```python
from build123d import *

# Parameters (mm, degrees)
SKETCH1_W                = 7.9
SKETCH1_H                = 95.7
BOSS_EXTRUDE1_DEPTH      = 9.2
SKETCH1_3_W              = 7.9
SKETCH1_3_H              = 95.7
BOSS_EXTRUDE2_DEPTH      = 9.2
BOSS_EXTRUDE3_DEPTH      = 32
BOSS_EXTRUDE3_DEPTH_BACK = 16
SKETCH2_R                = 3.8
BOSS_EXTRUDE4_DEPTH      = 0.0001
BOSS_EXTRUDE4_DEPTH_BACK = 6
SKETCH4_R                = 0.5


with BuildPart() as part:
    # Sketch1 → Boss-Extrude1 (new body)
    with BuildSketch(Plane(origin=(0, 0, 0), x_dir=(0, 0, -1), z_dir=(1, 0, 0))):
        with Locations((-28.171698113, -0.670754717)):
            Rectangle(SKETCH1_W, SKETCH1_H)
    extrude(amount=BOSS_EXTRUDE1_DEPTH)

    # Sketch1_3 → Boss-Extrude2 (add)
    with BuildSketch(Plane(origin=(0, 0, 0), x_dir=(0, 0, -1), z_dir=(1, 0, 0))):
        with Locations((-28.171698113, -0.670754717)):
            Rectangle(SKETCH1_3_W, SKETCH1_3_H)
        with Locations((-4.071698113, -0.670754717)):
            Rectangle(SKETCH1_3_W, SKETCH1_3_H)
    extrude(amount=BOSS_EXTRUDE2_DEPTH)


with BuildPart() as boss_extrude2_piece_1:
    # of the separate pieces the step leaves, piece 1, a body of its own (boss_extrude2_pieces)
    add(part.part.solids().sort_by_distance((0, 47.179245283, 8.021698113))[0])



with BuildPart() as boss_extrude2_piece_2:
    # of the separate pieces the step leaves, piece 2, a body of its own (boss_extrude2_pieces)
    add(part.part.solids().sort_by_distance((0, 47.179245283, 32.121698113))[0])


with BuildPart() as boss_extrude2_piece_1_1:
    add(boss_extrude2_piece_1.part)

    add(boss_extrude2_piece_2.part)  # Boss-Extrude3 merges Boss-Extrude2 piece 2
    # Sketch2 → Boss-Extrude3 (add, two sides: drawn at the far end of the back side and taken through both)
    with BuildSketch(Plane.XY.offset(8.021698113).offset(-BOSS_EXTRUDE3_DEPTH_BACK)):
        with Locations(Location((4.3, 30.179245283, 0), (0, 0, 90))):
            Circle(SKETCH2_R)
    extrude(amount=BOSS_EXTRUDE3_DEPTH + BOSS_EXTRUDE3_DEPTH_BACK)

    # Sketch4 → Boss-Extrude4 (add, two sides: drawn at the far end of the back side and taken through both)
    with BuildSketch(Plane(origin=(9.2, 0, 0), x_dir=(0, 0, -1), z_dir=(1, 0, 0)).offset(-BOSS_EXTRUDE4_DEPTH_BACK)):
        with Locations((-16.121698113, 30.179245283)):
            Circle(SKETCH4_R)
    extrude(amount=BOSS_EXTRUDE4_DEPTH + BOSS_EXTRUDE4_DEPTH_BACK)


solid = boss_extrude2_piece_1_1.part
```
Verification items for the finished model (mm, model axes). A direction names the side the tool comes from. Coordinates: 2 decimals unless noted, no trailing zeros. Order: outer loops, then holes, each group sorted by start corner. A loop starts at its lowest first (then second) coordinate and runs counter-clockwise, first axis right, second up. Notation, with made-up numbers: (59.25, 59) - (74.25, 59) arc R19 ccw to (74.25, 75) - close; hole circle Ø5 at (4, 21.25). An arc over 180 degrees is marked (long way). Return JSON: item names as keys, results as strings.
(1) Section check B-B, the plane x = 4.3. Record the cut outline in (y, z).
Filled sheet:
{"outline": "(-48.52, 0.12) - (26.38, 0.12) - (26.38, -7.98) - (33.98, -7.98) - (33.98, 0.12) - (47.18, 0.12) - (47.18, 8.02) - (33.98, 8.02) - (33.98, 24.22) - (47.18, 24.22) - (47.18, 32.12) - (33.98, 32.12) - (33.98, 40.02) - (26.38, 40.02) - (26.38, 32.12) - (-48.52, 32.12) - (-48.52, 24.22) - (26.38, 24.22) - (26.38, 8.02) - (-48.52, 8.02) - close"}
(2) Section check A-A, the plane y = 37.5. Record the cut outline in (x, z), and give its area (3 significant figures).
Filled sheet:
{"outline": "(0, 0.12) - (9.2, 0.12) - (9.2, 8.02) - (0, 8.02) - close; (0, 24.22) - (9.2, 24.22) - (9.2, 32.12) - (0, 32.12) - close", "area": "145 mm^2"}
(3) Access from +Z, -Z, +X, -X, +Y, -Y to the whole of each face (thin tool, end or side, straight path). Record for faces 5 (the cylindrical face through (4.133, 26.383, 36.016)), 6 (the flat face through (5, 47.179, 28)), 7 (the cylindrical face through (4.133, 26.383, -3.985)).
Filled sheet:
{"face 5": "+Z", "face 6": "+Z, -Z, +X, -X, +Y", "face 7": "-Z"}
(4) Section check C-C, the plane z = 20. Record the cut outline in (x, y), and give its area (3 significant figures).
Filled sheet:
{"outline": "circle Ø7.6 at (4.3, 30.18)", "area": "45.4 mm^2"}
(5) Mould release check, pull along Z, two halves, no side actions. Record for faces 1 (the flat face through (5, -1, 0.122)), 2 (the cylindrical face through (4.133, 26.383, 16.008)), 3 (the flat face through (5, -1, 24.222)), 4 (the flat face through (5, -48.521, 4)): pulls with the +Z half, pulls with the -Z half, needs draft (parallel to the pull), parting line crosses it, or undercut.
Filled sheet:
{"face 1": "pulls with the -Z half", "face 2": "undercut", "face 3": "undercut", "face 4": "needs draft"}
(6) Go/stop test with flat-tipped pins: pin 1 (1 mm diameter, centred on x = 5, z = 18.5, fed in from +Y); pin 2 (3 mm diameter, centred on x = 3.5, y = -32.5, fed in from -Z); pin 3 (4.5 mm diameter, centred on x = 3, y = -9, fed in from +Z); pin 4 (12 mm diameter, centred on y = 22, z = -3, fed in from +X). Record where each tip stops, or that it passes through.
Filled sheet:
{"pin 1": "stops at y = 33.97", "pin 2": "stops at z = 0.12", "pin 3": "stops at z = 32.12", "pin 4": "stops at x = 9.2"}
(7) Thickness scan on line 1 along Z through (x, y) = (4.5, -26); line 2 along Y through (x, z) = (6.5, 15); line 3 along Y through (x, z) = (4.75, 13). Record the ranges inside material, lowest first.
Filled sheet:
{"line 1": "z = 0.12 to 8.02, 24.22 to 32.12", "line 2": "y = 27.08 to 33.28", "line 3": "y = 26.41 to 33.95"}
